The model under review builds one solid part; all positions refer to its coordinate system, in mm. Face numbers are marked on the shaded views. Round coordinates to 2 decimals unless told otherwise and drop trailing zeros. Write each loop counter-clockwise with the first axis right and the second up, starting at its lowest first coordinate (ties: lowest second). Pieces come first, ordered by that corner, then holes. Notation, with made-up numbers: (36.25, 1) - (70.25, 1) arc R14 ccw to (70.25, 16) - close; hole circle Ø4 at (83, 3). An arc over 180 degrees is marked (long way). Return JSON: item names as keys, results as strings.
from build123d import *

# Parameters (mm, degrees)
SKETCH_1_W          = 82
SKETCH_1_H          = 82
SKETCH_1_R          = 35.5
EXTRUDE_1_DEPTH     = 245
SKETCH_2_W          = 82
SKETCH_2_H          = 82
EXTRUDE_2_DEPTH     = 27
SKETCH_3_W          = 8
SKETCH_3_H          = 20
CUT_EXTRUDE_1_DEPTH = 245
SKETCH_4_R          = 4
CUT_EXTRUDE_2_DEPTH = 20
FILLET_2_R          = 3
FILLET_3_R          = 3
FILLET_4_R          = 3
FILLET_5_R          = 3
SKETCH_5_R          = 1.05
CUT_EXTRUDE_3_DEPTH = 10
EXTRUDE_START       = 0.2
SKETCH_6_R          = 1.05
EXTRUDE_3_DEPTH     = 0.2
CUT_EXTRUDE_5_REACH = 263.591
SKETCH_7_W          = 20
SKETCH_7_H          = 65
CUT_EXTRUDE_6_REACH = 263.591
SKETCH_8_W          = 41
SKETCH_8_H          = 20
SKETCH_9_R          = 1.2
CUT_EXTRUDE_7_DEPTH = 10


with BuildPart() as part:
    # 草圖1 → 填料-伸長1 (new body)
    with BuildSketch(Plane.XY):
        Rectangle(SKETCH_1_W, SKETCH_1_H)
        Circle(SKETCH_1_R, mode=Mode.SUBTRACT)
    extrude(amount=EXTRUDE_1_DEPTH)

    # 草圖2 → 填料-伸長2 (add)
    with BuildSketch(Plane(origin=(0, 0, 0), x_dir=(-1, 0, 0), z_dir=(0, 0, -1))):
        Rectangle(SKETCH_2_W, SKETCH_2_H)
    extrude(amount=EXTRUDE_2_DEPTH)

    # 草圖3 → 除料-伸長1 (cut)
    with BuildSketch(Plane.XY.offset(245)):
        with Locations((-37, 0)):
            Rectangle(SKETCH_3_W, SKETCH_3_H)
    extrude(amount=-CUT_EXTRUDE_1_DEPTH, mode=Mode.SUBTRACT)

    # 草圖4 → 除料-伸長2 (cut)
    with BuildSketch(Plane.XY.offset(245)):
        with Locations((-32.9, 33)):
            Circle(SKETCH_4_R)
        with Locations((33.1, 32.9)):
            Circle(SKETCH_4_R)
        with Locations((33, -33.1)):
            Circle(SKETCH_4_R)
        with Locations((-33, -33)):
            Circle(SKETCH_4_R)
    extrude(amount=-CUT_EXTRUDE_2_DEPTH, mode=Mode.SUBTRACT)

    # 圓角2
    fillet_2_edges = [part.edges().sort_by_distance(p)[0] for p in [
        (-36.9, 33, 225),
    ]]
    fillet(fillet_2_edges, radius=FILLET_2_R)

    # 圓角3
    fillet_3_edges = [part.edges().sort_by_distance(p)[0] for p in [
        (29.1, 32.9, 225),
    ]]
    fillet(fillet_3_edges, radius=FILLET_3_R)

    # 圓角4
    fillet_4_edges = [part.edges().sort_by_distance(p)[0] for p in [
        (-37, -33, 225),
    ]]
    fillet(fillet_4_edges, radius=FILLET_4_R)

    # 圓角5
    fillet_5_edges = [part.edges().sort_by_distance(p)[0] for p in [
        (29, -33.1, 225),
    ]]
    fillet(fillet_5_edges, radius=FILLET_5_R)

    # 草圖5 → 除料-伸長3 (cut)
    with BuildSketch(Plane(origin=(0, 41, 0), x_dir=(1, 0, 0), z_dir=(0, 1, 0))):
        with Locations(Location((-36.75, 22.75, 0), (0, 0, 270))):
            Circle(SKETCH_5_R)
        with Locations(Location((-36.75, 4.75, 0), (0, 0, 270))):
            Circle(SKETCH_5_R)
    extrude(amount=-CUT_EXTRUDE_3_DEPTH, mode=Mode.SUBTRACT)

    # 草圖6 → 填料-伸長3 (add)
    with BuildSketch(Plane(origin=(0, 35, 0), x_dir=(1, 0, 0), z_dir=(0, 1, 0)).offset(EXTRUDE_START)):
        with Locations(Location((-36.75, 22.75, 0), (0, 0, 270))):
            Circle(SKETCH_6_R)
        with Locations(Location((-36.75, 4.75, 0), (0, 0, 270))):
            Circle(SKETCH_6_R)
    extrude(amount=-EXTRUDE_3_DEPTH)

    # 草圖7 → 除料-伸長5 (cut, up to next)
    with BuildSketch(Plane(origin=(-41, 0, 0), x_dir=(0, 0, -1), z_dir=(1, 0, 0)), mode=Mode.PRIVATE) as cut_extrude_5_sk1:
        with Locations((17, -8.5)):
            Rectangle(SKETCH_7_W, SKETCH_7_H)
    cut_extrude_5_tool1 = extrude(cut_extrude_5_sk1.sketch, amount=CUT_EXTRUDE_5_REACH, mode=Mode.PRIVATE) & part.part
    add(cut_extrude_5_tool1.solids().sort_by_distance((-41, -8.5, -17))[0], mode=Mode.SUBTRACT)

    # 草圖8 → 除料-伸長6 (cut, up to next)
    with BuildSketch(Plane(origin=(0, 41, 0), x_dir=(1, 0, 0), z_dir=(0, 1, 0)), mode=Mode.PRIVATE) as cut_extrude_6_sk1:
        with Locations((20.5, 17)):
            Rectangle(SKETCH_8_W, SKETCH_8_H)
    cut_extrude_6_tool1 = extrude(cut_extrude_6_sk1.sketch, amount=-CUT_EXTRUDE_6_REACH, mode=Mode.PRIVATE) & part.part
    add(cut_extrude_6_tool1.solids().sort_by_distance((20.5, 41, -17))[0], mode=Mode.SUBTRACT)

    # 草圖9 → 除料-伸長7 (cut)
    with BuildSketch(Plane(origin=(0, 0, -7), x_dir=(-1, 0, 0), z_dir=(0, 0, -1))):
        with Locations((-33, 33)):
            Circle(SKETCH_9_R)
        with Locations((-33, -33)):
            Circle(SKETCH_9_R)
        with Locations((33, -33)):
            Circle(SKETCH_9_R)
        with Locations((38, 20)):
            Circle(SKETCH_9_R)
    extrude(amount=-CUT_EXTRUDE_7_DEPTH, mode=Mode.SUBTRACT)


solid = part.part
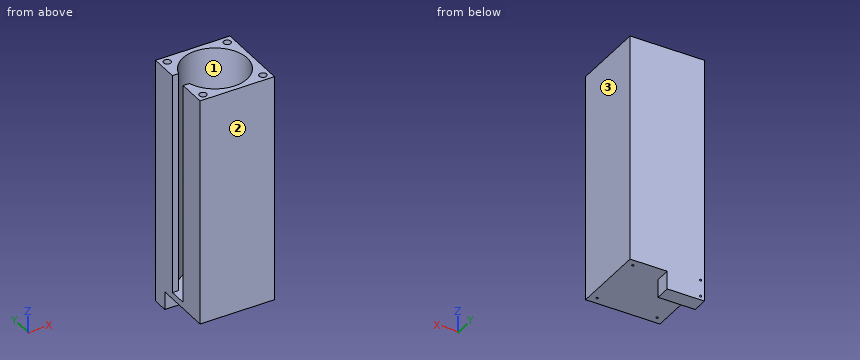
(1) Wall thickness on line 1 (Y direction, x = 0.5, z = 40); line 2 (X direction, y = 15.5, z = 79); line 3 (Y direction, x = -33, z = -1): over which ranges is each line inside the solid? List them lowest first.
Filled in:
{"line 1": "y = -41 to -35.5, 35.5 to 41", "line 2": "x = -41 to -31.94, 31.94 to 41", "line 3": "y = -41 to -34.2, -31.8 to 41"}
(2) Add section A-A (z = 17.5). Write out the cut boundary in (x, y), plus the area to 3 significant figures.
Filled in:
{"outline": "(-41, -41) - (41, -41) - (41, 41) - (-41, 41) - (-41, 10) - (-34.06, 10) arc R35.5 cw (long way) to (-34.06, -10) - (-41, -10) - close", "area": "2,650 mm2"}
(3) Add section D-D (x = 25). Write out the cut boundary in (y, z).
Filled in:
{"outline": "(-41, -7) - (41, -7) - (41, 245) - (25.2, 245) - (25.2, 0) - (-25.2, 0) - (-25.2, 245) - (-41, 245) - close"}
(4) Add section C-C (x = -16). Write out the cut boundary in (y, z).
Filled in:
{"outline": "(-41, -7) - (24, -7) - (24, -27) - (41, -27) - (41, 245) - (31.69, 245) - (31.69, 0) - (-31.69, 0) - (-31.69, 245) - (-41, 245) - close"}
(5) Clearance check with flat-ended pins moving along their axes: pin 1 Ø3 at (x, y) = (15.5, -12.5) entering from +Z; pin 2 Ø1.6 at (x, y) = (-33.5, 33) entering from +Z; pin 3 Ø1.7 at (x, z) = (-36.5, -23) entering from +Y; pin 4 Ø4 at (x, y) = (33, 33) entering from +Z. State where each tip first meets the part, or that it passes through.
Filled in:
{"pin 1": "stops at z = 0", "pin 2": "stops at z = 225.03", "pin 3": "stops at y = 41", "pin 4": "stops at z = 225.23"}
(6) Mouldability with a two-part tool opening along X and no side actions: class the marked faces 1, 2 and 3 as released by +X, released by -X, zero draft, split by the parting line, or undercut.
Filled in:
{"face 1": "undercut", "face 2": "zero draft", "face 3": "released by +X"}
(7) Add section B-B (y = 0). Write out the cut boundary in (x, z).
Filled in:
{"outline": "(-41, -7) - (41, -7) - (41, 245) - (35.5, 245) - (35.5, 0) - (-41, 0) - close"}
